```python
from build123d import *

# Parameters (mm, degrees)
BOSS_EXTRUDE1_DEPTH = 20
BOSS_EXTRUDE2_DEPTH = 3
SKETCH4_W           = 10
SKETCH4_H           = 10
BOSS_EXTRUDE3_DEPTH = 17
SKETCH5_R           = 3
BOSS_EXTRUDE4_DEPTH = 20
SKETCH6_W           = 5
SKETCH6_H           = 9
CUT_EXTRUDE1_DEPTH  = 30
SKETCH7_W           = 58
SKETCH7_H           = 32
SKETCH7_W_2         = 52
SKETCH7_H_2         = 26
BOSS_EXTRUDE5_DEPTH = 5


with BuildPart() as part:
    # Sketch1 → Boss-Extrude1 (new body)
    with BuildSketch(Plane.XY):
        with BuildLine():
            Line((-25, 75.5), (25, 75.5))
            ThreePointArc((25, 75.5), (34.192388155, 71.692388155), (38, 62.5))
            Line((38, 62.5), (38, -62.5))
            ThreePointArc((38, -62.5), (34.192388155, -71.692388155), (25, -75.5))
            Line((25, -75.5), (-25, -75.5))
            ThreePointArc((-25, -75.5), (-34.192388155, -71.692388155), (-38, -62.5))
            Line((-38, -62.5), (-38, 62.5))
            ThreePointArc((-38, 62.5), (-34.192388155, 71.692388155), (-25, 75.5))
        make_face()
        with BuildLine():
            Line((-25, 72.5), (25, 72.5))
            ThreePointArc((25, 72.5), (32.071067812, 69.571067812), (35, 62.5))
            Line((35, 62.5), (35, -62.5))
            ThreePointArc((35, -62.5), (32.071067812, -69.571067812), (25, -72.5))
            Line((25, -72.5), (-25, -72.5))
            ThreePointArc((-25, -72.5), (-32.071067812, -69.571067812), (-35, -62.5))
            Line((-35, -62.5), (-35, 62.5))
            ThreePointArc((-35, 62.5), (-32.071067812, 69.571067812), (-25, 72.5))
        make_face(mode=Mode.SUBTRACT)
    extrude(amount=BOSS_EXTRUDE1_DEPTH)

    # Sketch3 → Boss-Extrude2 (add)
    with BuildSketch(Plane(origin=(0, 0, 0), x_dir=(-1, 0, 0), z_dir=(0, 0, -1))):
        with BuildLine():
            Line((25, -75.5), (-25, -75.5))
            ThreePointArc((-25, -75.5), (-34.192388155, -71.692388155), (-38, -62.5))
            Line((-38, -62.5), (-38, 62.5))
            ThreePointArc((-38, 62.5), (-34.192388155, 71.692388155), (-25, 75.5))
            Line((-25, 75.5), (25, 75.5))
            ThreePointArc((25, 75.5), (34.192388155, 71.692388155), (38, 62.5))
            Line((38, 62.5), (38, -62.5))
            ThreePointArc((38, -62.5), (34.192388155, -71.692388155), (25, -75.5))
        make_face()
    extrude(amount=-BOSS_EXTRUDE2_DEPTH)

    # Sketch4 → Boss-Extrude3 (add)
    with BuildSketch(Plane.XY.offset(3)):
        with Locations((-25, 62.5)):
            Rectangle(SKETCH4_W, SKETCH4_H)
        with Locations((25, 62.5)):
            Rectangle(SKETCH4_W, SKETCH4_H)
        with Locations((25, -62.5)):
            Rectangle(SKETCH4_W, SKETCH4_H)
        with Locations((-25, -62.5)):
            Rectangle(SKETCH4_W, SKETCH4_H)
    extrude(amount=BOSS_EXTRUDE3_DEPTH)

    # Sketch5 → Boss-Extrude4 (add)
    with BuildSketch(Plane.XY.offset(20)):
        with Locations((-25, 62.5)):
            Circle(SKETCH5_R)
        with Locations(Location((25, 62.5, 0), (0, 0, 180))):
            Circle(SKETCH5_R)
        with Locations((25, -62.5)):
            Circle(SKETCH5_R)
        with Locations(Location((-25, -62.5, 0), (0, 0, 180))):
            Circle(SKETCH5_R)
    extrude(amount=BOSS_EXTRUDE4_DEPTH)

    # Sketch6 → Cut-Extrude1 (cut)
    with BuildSketch(Plane(origin=(38, 0, 0), x_dir=(0, 0, -1), z_dir=(1, 0, 0))):
        with Locations((-7.5, -29)):
            Rectangle(SKETCH6_W, SKETCH6_H)
        with Locations((-7.5, -78)):
            Rectangle(SKETCH6_W, SKETCH6_H)
    extrude(amount=-CUT_EXTRUDE1_DEPTH, mode=Mode.SUBTRACT)

    # Sketch7 → Boss-Extrude5 (add)
    with BuildSketch(Plane.XY.offset(3)):
        with Locations((9, 0)):
            Rectangle(SKETCH7_W, SKETCH7_H)
        with Locations((9, 0)):
            Rectangle(SKETCH7_W_2, SKETCH7_H_2, mode=Mode.SUBTRACT)
    extrude(amount=BOSS_EXTRUDE5_DEPTH)


solid = part.part
```
Geometry: final body of the model. Coordinates: model frame, mm. A direction names the side the tool comes from. Round coordinates to 2 decimals unless told otherwise and drop trailing zeros. Order: outer loops, then holes, each group sorted by start corner. A loop starts at its lowest first (then second) coordinate and runs counter-clockwise, first axis right, second up. Notation, with made-up numbers: (-39, 38) -> (2, 38) arc R17 ccw to (2, 54) -> close; hole circle Ø8 at (34.5, -1.75). An arc over 180 degrees is marked (long way). Use CSV: the item, a comma, the result in double quotes. Start each with the question number.
1) Section D-D (z = 29.5). Return the cut outline in (x, y).
2) Draft query along Y for faces 1 (the face through (20, 62, 11)), 2 (the face through (20, -73.5, 8)), 3 (the face through (31.99, 69.65, 11.38)), 4 (the face through (1, 1, 0)). Return one class per face: +Y half, -Y half, draft (parallel to the pull), parting line (faces both ways), or undercut.
3) Section B-B (y = 49.5). Return the cut outline in (x, z), and give its area (3 significant figures).
4) Set-up query: faces 5 (the face through (0, -75.5, 10)), 6 (the face through (-22.79, -64.53, 29.86)). Return all of +Z, -Z, +X, -X, +Y, -Y with unobstructed straight access to the full face (end or side cutting, diameter ignored); none if empty.
5) Section C-C (x = -23.5). Return the cut outline in (y, z).
6) Material intervals for line 1 along Y through (x, z) = (15, 7); line 2 along Y through (x, z) = (-9.5, 4); line 3 along Y through (x, z) = (21.5, 6.5), sorted ascending. Write a range as from..to.
7) First-contact query: pin 1 Ø2.5 at (x, z) = (36.5, 6.5) entering from -Y; pin 2 Ø1.5 at (x, z) = (-26, 22.5) entering from -Y; pin 3 Ø5 at (x, y) = (-13, 54.5) entering from +Z. Flat tips, straight axial feed; report the tip coordinate or a pass-through.
8) Section A-A (z = 13). State how many separate pieces and enclosed holes the cut face has, and give its area (3 significant figures).
Returned:
1,outline,"circle Ø6 at (-25, -62.5); circle Ø6 at (-25, 62.5); circle Ø6 at (25, -62.5); circle Ø6 at (25, 62.5)"
2,face 1,"undercut"
2,face 2,"-Y half"
2,face 3,"undercut"
2,face 4,"draft"
3,outline,"(-38, 0) -> (38, 0) -> (38, 20) -> (35, 20) -> (35, 3) -> (-35, 3) -> (-35, 20) -> (-38, 20) -> close"
3,area,"330 mm²"
4,face 5,"+Z, -Z, +X, -X, -Y"
4,face 6,"+Z"
5,outline,"(-75.5, 0) -> (75.5, 0) -> (75.5, 20) -> (72.5, 20) -> (72.5, 3) -> (67.5, 3) -> (67.5, 20) -> (65.1, 20) -> (65.1, 40) -> (59.9, 40) -> (59.9, 20) -> (57.5, 20) -> (57.5, 3) -> (-57.5, 3) -> (-57.5, 20) -> (-59.9, 20) -> (-59.9, 40) -> (-65.1, 40) -> (-65.1, 20) -> (-67.5, 20) -> (-67.5, 3) -> (-72.5, 3) -> (-72.5, 20) -> (-75.5, 20) -> close"
6,line 1,"y = -73.5..-72.5, -16..-13, 13..16, 72.5..75.5"
6,line 2,"y = -75.5..-72.5, -16..-13, 13..16, 72.5..75.5"
6,line 3,"y = -73.5..-72.5, -67.5..-57.5, -16..-13, 13..16, 57.5..67.5, 72.5..75.5"
7,pin 1,"stops at y = -70.5"
7,pin 2,"stops at y = -65.49"
7,pin 3,"stops at z = 3"
8,separate pieces,"5"
8,enclosed holes,"1"
8,area,"1,670 mm²"
